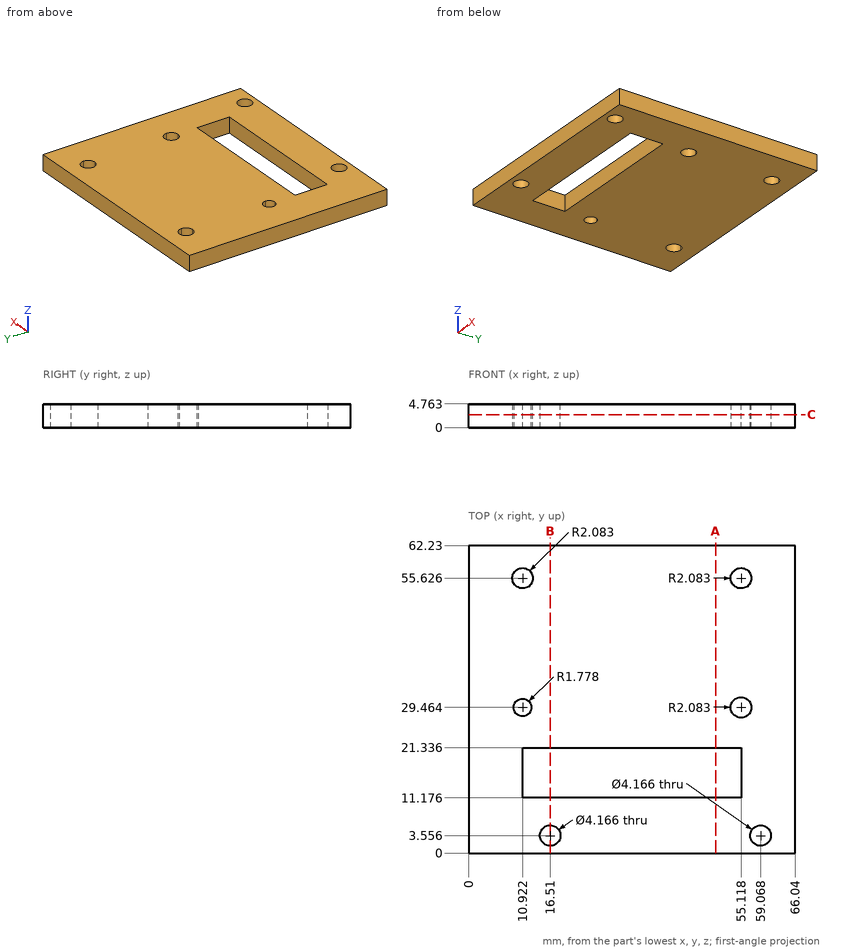
Job drawing, mm, ordinate dimensions from the low corner. One solid piece. Coordinates: 2 decimals unless noted, no trailing zeros. Order: outer loops, then holes, each group sorted by start corner. A loop starts at its lowest first (then second) coordinate and runs counter-clockwise, first axis right, second up. Notation, with made-up numbers: (57.5, 60) -> (86.5, 60) arc R19 cw to (86.5, 93) -> close; hole circle Ø4 at (-13.75, -39.75). An arc over 180 degrees is marked (long way). Return JSON: item names as keys, results as strings. Group by question number.
Item 1: Saw through at B-B on x = 16.51. Write the cut outline in (y, z) (1 decimal).
Item 2: Wall check: line 1 along X through (y, z) = (29.5, 1.85) (1 decimal); line 2 along Y through (x, z) = (16.51, 3.8) (1 decimal); line 3 along Y through (x, z) = (55, 2.7) (1 decimal). Give the ranges that are in metal, low to high. Write a range as [from, to].
Item 3: Saw through at C-C on z = 2.6. Write the cut outline in (x, y) (1 decimal).
Item 4: Flat gauge pins, fed straight in: P1, Ø1, axis at x = 30, z = 2, coming from the -Y side; P2, Ø1, axis at x = 44.5, y = 13.5, coming from the +Z side. Where does each tip first touch, or does it go through?
Item 5: Saw through at A-A on x = 50. Write the cut outline in (y, z) (1 decimal), then the cut area to 3 significant figures.
Values found:
{
 "1": {"outline": "(0, 0) -> (1.5, 0) -> (1.5, 4.8) -> (0, 4.8) -> close; (5.6, 0) -> (11.2, 0) -> (11.2, 4.8) -> (5.6, 4.8) -> close; (21.3, 0) -> (62.2, 0) -> (62.2, 4.8) -> (21.3, 4.8) -> close"},
 "2": {"line 1": "x = [0, 9.1], [12.7, 53], [57.2, 66]", "line 2": "y = [0, 1.5], [5.6, 11.2], [21.3, 62.2]", "line 3": "y = [0, 11.2], [21.3, 27.4], [31.5, 53.5], [57.7, 62.2]"},
 "3": {"outline": "(0, 0) -> (66, 0) -> (66, 62.2) -> (0, 62.2) -> close; hole circle Ø4.2 at (10.9, 55.6); hole circle Ø3.6 at (10.9, 29.5); hole (10.9, 11.2) -> (55.1, 11.2) -> (55.1, 21.3) -> (10.9, 21.3) -> close; hole circle Ø4.2 at (16.5, 3.6); hole circle Ø4.2 at (55.1, 29.5); hole circle Ø4.2 at (55.1, 55.6); hole circle Ø4.2 at (59.1, 3.6)"},
 "4": {"P1": "stops at y = 0", "P2": "passes through"},
 "5": {"outline": "(0, 0) -> (11.2, 0) -> (11.2, 4.8) -> (0, 4.8) -> close; (21.3, 0) -> (62.2, 0) -> (62.2, 4.8) -> (21.3, 4.8) -> close", "area": "248 mm2"}
}
